from build123d import *

# Parameters (mm, degrees)
SKETCH_1_R          = 5
EXTRUDE_1_DEPTH     = 4
SKETCH_2_R          = 3.6
EXTRUDE_2_DEPTH     = 0.3
FILLET_1_R          = 2
SKETCH_3_R          = 0.6
CUT_EXTRUDE_1_DEPTH = 9.275868534


with BuildPart() as part:
    # 草图1 → 凸台-拉伸1 (new body)
    with BuildSketch(Plane(origin=(0, 0, 0), x_dir=(1, 0, 0), z_dir=(0, 1, 0))):
        with Locations(Location((0, 0, 0), (0, 0, 270))):
            Circle(SKETCH_1_R)
    extrude(amount=EXTRUDE_1_DEPTH)

    # 草图2 → 凸台-拉伸2 (add)
    with BuildSketch(Plane(origin=(0, 4, 0), x_dir=(1, 0, 0), z_dir=(0, 1, 0))):
        with Locations(Location((0, 0, 0), (0, 0, 270))):
            Circle(SKETCH_2_R)
    extrude(amount=EXTRUDE_2_DEPTH)

    # 圆角1
    fillet_1_edges = [part.edges().sort_by_distance(p)[0] for p in [
        (0, 0, -5),
    ]]
    fillet(fillet_1_edges, radius=FILLET_1_R)

    # 草图3 → 切除-拉伸1 (cut, through all)
    with BuildSketch(Plane(origin=(0, 4.3, 0), x_dir=(1, 0, 0), z_dir=(0, 1, 0))):
        with Locations(Location((0, 0, 0), (0, 0, 270))):
            Circle(SKETCH_3_R)
    extrude(amount=-CUT_EXTRUDE_1_DEPTH, mode=Mode.SUBTRACT)


solid = part.part
Verification items for the finished model (mm, model axes). A direction names the side the tool comes from. Coordinates: 2 decimals unless noted, no trailing zeros. Write each loop counter-clockwise with the first axis right and the second up, starting at its lowest first coordinate (ties: lowest second). Pieces come first, ordered by that corner, then holes. Notation, with made-up numbers: M 43,58 L 73,58 A14 ccw 73,84 Z; hole C -34.75,62.25 d4. An arc over 180 degrees is marked long. Use CSV: the item, a comma, the result in double quotes.
Q1. Mould release check, pull along X, two halves, no side actions. Record for faces 3 (the flat face through (0, 0, 1)), 4 (the cylindrical face through (0.506, 2.18, 0.323)), 5 (the cylindrical face through (-4.88, 2.99, -1.08)): pulls with the +X half, pulls with the -X half, needs draft (parallel to the pull), parting line crosses it, or undercut.
Computed values:
face 3,"needs draft"
face 4,"undercut"
face 5,"parting line crosses it"
Q2. Section check C-C, the plane y = 0.8. Enter the section's corners in (x, z).
Computed values:
outline,"C 0,0 d9.2; hole C 0,0 d1.2"
Q3. Section check D-D, the plane y = 2.9. Enter the section's corners in (x, z), and give its area (3 significant figures).
Computed values:
outline,"C 0,0 d10; hole C 0,0 d1.2"
area,"77.4 mm²"
Q4. Set-up check for faces 1 (the flat face through (-1, 4.3, 0)), 2 (the flat face through (-3.3, 4, 2.2)): record each of +Z, -Z, +X, -X, +Y, -Y from which the full face is reachable in a straight line by a thin tool's end or side.
Computed values:
face 1,"+Z, -Z, +X, -X, +Y"
face 2,"+Y"
Q5. Thickness scan on line 1 along Z through (x, y) = (-0.5, 1); line 2 along X through (y, z) = (1.3, 0); line 3 along Y through (x, z) = (-3.5, 1.25). Record the ranges inside material, lowest first. Write a range as [from, to].
Computed values:
line 1,"[-4.71, -0.33], [0.33, 4.71]"
line 2,"[-4.87, -0.6], [0.6, 4.87]"
line 3,"[0.13, 4]"
Q6. Section check A-A, the plane x = 0. Enter the section's corners in (y, z).
Computed values:
outline,"M 0,-3 A2 ccw 2,-5 L 4,-5 L 4,-3.6 L 4.3,-3.6 L 4.3,-0.6 L 0,-0.6 Z; M 0,0.6 L 4.3,0.6 L 4.3,3.6 L 4,3.6 L 4,5 L 2,5 A2 ccw 0,3 Z"
Q7. Section check B-B, the plane z = 0. Enter the section's corners in (x, y), and give its area (3 significant figures).
Computed values:
outline,"M -5,2 A2 ccw -3,0 L -0.6,0 L -0.6,4.3 L -3.6,4.3 L -3.6,4 L -5,4 Z; M 0.6,0 L 3,0 A2 ccw 5,2 L 5,4 L 3.6,4 L 3.6,4.3 L 0.6,4.3 Z"
area,"35.3 mm²"
